Study the drawing (mm; zero at the part's minimum x, y, z) and answer. Coordinates: 2 decimals unless noted, no trailing zeros. Order: outer loops, then holes, each group sorted by start corner. A loop starts at its lowest first (then second) coordinate and runs counter-clockwise, first axis right, second up. Notation, with made-up numbers: M 57,5.25 L 73,5.25 A16 cw 73,33.25 Z; hole C -34,14.5 d4. An arc over 180 degrees is marked long. Use a Markdown table: item, result. Add a question column.
1) Find section A-A on y = 39. Write down the section's boundary in (x, z).
2) Find section C-C on z = 31.5. Write down the section's boundary in (x, y).
3) Find section D-D on x = 23.5. Write down the section's boundary in (y, z), plus the area to 3 significant figures.
4) The mould has two halves that part along Y. Classify the marked faces 1, 2 and 3: released by +Y, released by -Y, zero draft, split by the parting line, or undercut.
5) Each of these flat-tipped pins is pushed along its axis until it touches: pin 1 Ø6 at (x, z) = (10.5, 9.5) entering from +Y; pin 2 Ø3 at (x, z) = (61.5, 19.5) entering from -Y; pin 3 Ø6 at (x, z) = (35.5, 10) entering from -Y. Where does it stop, or does it pass through?
6) Find the intervals of material crossed by probe 1 along Y at (x, z) = (39, 13); probe 2 along Z at (x, y) = (72.5, 54); probe 3 along Y at (x, z) = (35, 20.5), in increasing order. Write a range as [from, to].
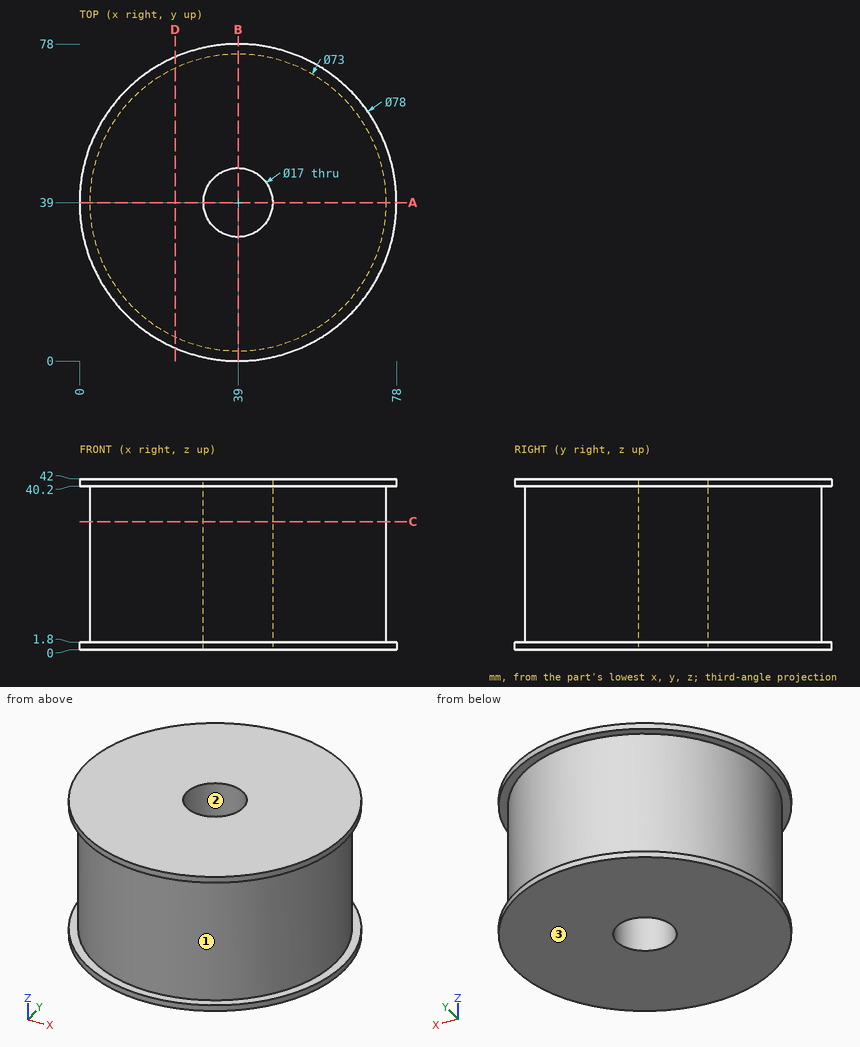
Check result:
| question | item | result |
|---|---|---|
| 1 | outline | M 0,0 L 30.5,0 L 30.5,42 L 0,42 L 0,40.2 L 2.5,40.2 L 2.5,1.8 L 0,1.8 Z; M 47.5,0 L 78,0 L 78,1.8 L 75.5,1.8 L 75.5,40.2 L 78,40.2 L 78,42 L 47.5,42 Z |
| 2 | outline | C 39,39 d73; hole C 39,39 d17 |
| 3 | outline | M 3.21,0 L 74.79,0 L 74.79,1.8 L 72.05,1.8 L 72.05,40.2 L 74.79,40.2 L 74.79,42 L 3.21,42 L 3.21,40.2 L 5.95,40.2 L 5.95,1.8 L 3.21,1.8 Z |
| 3 | area | 2,800 mm2 |
| 4 | face 1 | split by the parting line |
| 4 | face 2 | undercut |
| 4 | face 3 | zero draft |
| 5 | pin 1 | stops at y = 65.12 |
| 5 | pin 2 | stops at y = 9.15 |
| 5 | pin 3 | stops at y = 2.5 |
| 6 | probe 1 | y = [2.5, 30.5], [47.5, 75.5] |
| 6 | probe 2 | z = [0, 1.8], [40.2, 42] |
| 6 | probe 3 | y = [2.72, 31.5], [46.5, 75.28] |
